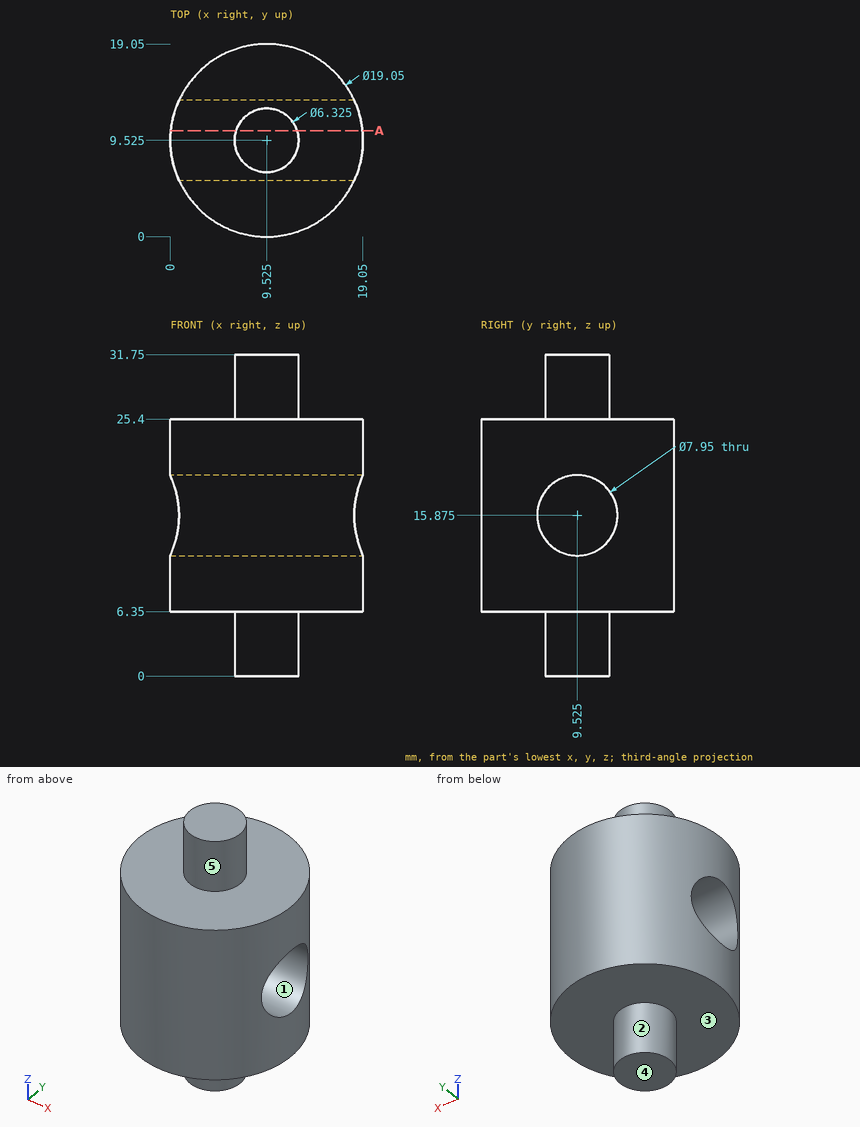
Source: three-view drawing plus pictorial views. Frame: mm from the lowest corner of the part. A direction names the side the tool comes from. Coordinates: 2 decimals unless noted, no trailing zeros. Loops run counter-clockwise (first coordinate to the right, second up) from the corner with the lowest first, then second, coordinate; pieces in that order, holes last. Notation, with made-up numbers: (54.5, 17) -> (77.5, 17) arc R21 cw to (77.5, 44) -> close; hole circle Ø7 at (51.5, 3.5). An arc over 180 degrees is marked (long way). Write each question's results on one line, items separated by ' | '. Start each with the question number.
Q1. Pin query (flat end, axial travel): pin 1 (8 mm diameter, centred on x = 4.5, z = 20, fed in from -Y) (1 decimal); pin 2 (4 mm diameter, centred on x = 7, z = 22.5, fed in from -Y); pin 3 (2 mm diameter, centred on x = 3.5, y = 4, fed in from -Z). Return the tip coordinate at first contact, or that it passes through.
Q2. Section A-A, the plane y = 10.5. Return the cut outline in (x, z), plus the area to 3 significant figures.
Q3. Pull-direction query (Y, two-part tool) for the marked faces 1, 2 and 3; classes: released by +Y, released by -Y, zero draft, split by the parting line, or undercut.
Q4. Ray query, line 1 (Z direction, x = 13.5, y = 5.5); line 2 (Y direction, x = 1.5, z = 18) (1 decimal); line 3 (Z direction, x = 9.75, y = 6.75). Return the intervals inside material, ascending. Write a range as from..to.
Q5. Reachability of the marked faces 4 and 5 from +Z, -Z, +X, -X, +Y, -Y: full face, straight path, thin tool, end or side. Return the list, or none.
Found:
1) pin 1: y = 0.1 | pin 2: y = 0.01 | pin 3: z = 6.35
2) outline: (0.05, 6.35) -> (6.52, 6.35) -> (6.52, 0) -> (12.53, 0) -> (12.53, 6.35) -> (19, 6.35) -> (19, 12.02) -> (0.05, 12.02) -> close; (0.05, 19.73) -> (19, 19.73) -> (19, 25.4) -> (12.53, 25.4) -> (12.53, 31.75) -> (6.52, 31.75) -> (6.52, 25.4) -> (0.05, 25.4) -> close | area: 291 mm2
3) face 1: undercut | face 2: split by the parting line | face 3: zero draft
4) line 1: 6.35..25.4 | line 2: 4.4..6.2, 12.9..14.7 | line 3: 0..13.03, 18.72..31.75
5) face 4: -Z, +X, -X, +Y, -Y | face 5: +Z
